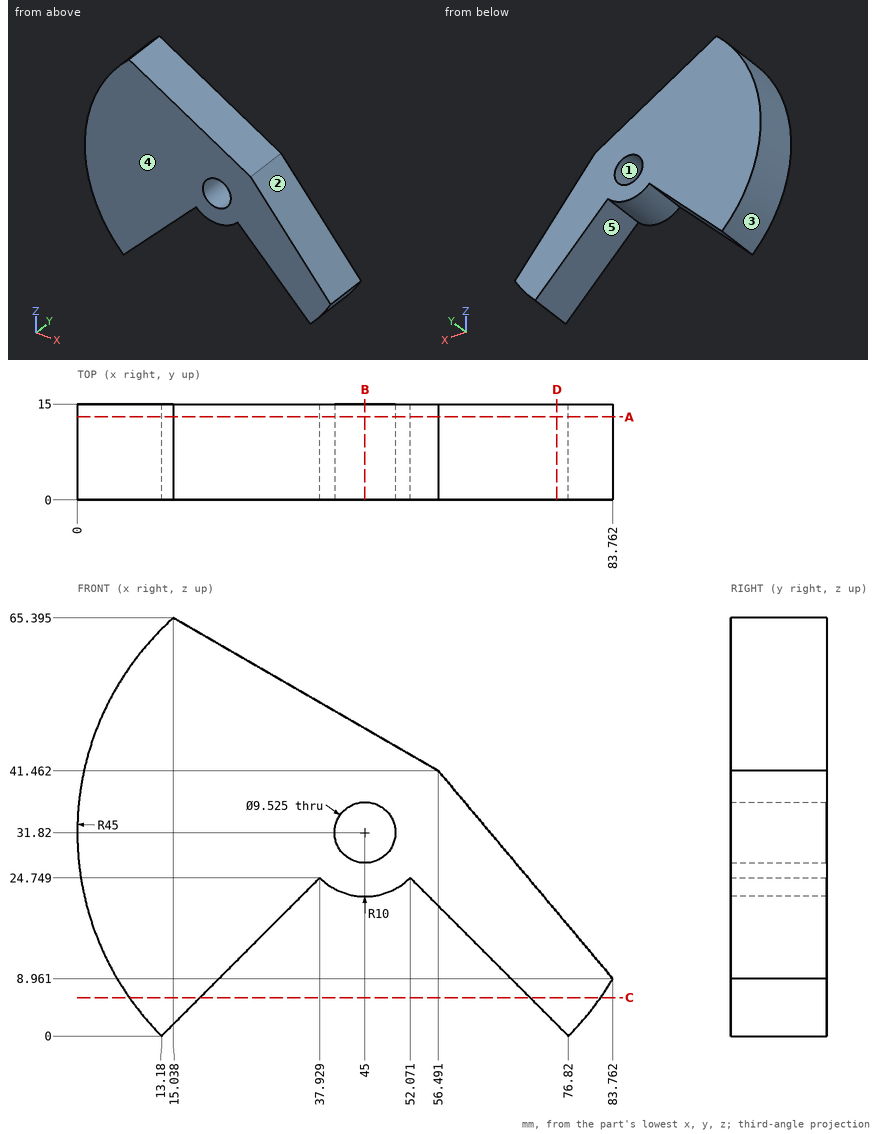
Could you check a few things on this drawing? It's one solid part, dimensions in mm from its lowest x, y, z. A direction names the side the tool comes from. Give positions to 0.01 mm unless a question says otherwise; leave off trailing zeros. Order: outer loops, then holes, each group sorted by start corner. A loop starts at its lowest first (then second) coordinate and runs counter-clockwise, first axis right, second up. Notation, with made-up numbers: M -17.75,17 L 32.25,17 A31 cw 32.25,44 Z; hole C 36.5,45 d1. An arc over 180 degrees is marked long. Use one line per item in the form item = value.
Item 1: If we section it at A-A, the plane y = 13: Write out the boundary of the cut face in (x, z) (1 decimal), and give its area (3 significant figures).
Values follow:
outline = M 13.2,0 L 37.9,24.7 A10 ccw 52.1,24.7 L 76.8,0 A45 ccw 83.8,9 L 56.5,41.5 L 15,65.4 A45 ccw Z; hole C 45,31.8 d9.5
area = 2,570 mm^2
Item 2: Thinking about a two-plate mould opening in X: for the marked faces 1, 2 and 3, which applies, pulls with the +X half, pulls with the -X half, needs draft (parallel to the pull), parting line crosses it, or undercut?
Values follow:
face_1 = undercut
face_2 = pulls with the +X half
face_3 = pulls with the -X half
Item 3: If we section it at D-D, the plane x = 75: Write out the boundary of the cut face in (y, z), and give its area (3 significant figures).
Values follow:
outline = M 0,1.82 L 15,1.82 L 15,19.4 L 0,19.4 Z
area = 264 mm^2
Item 4: Will these pins go through, and if not, where does the flat tip stop? pin 1 Ø3 at (x, y) = (31.5, 7) entering from +Z (1 decimal); pin 2 Ø5 at (y, z) = (5.5, 49.5) entering from +X (1 decimal); pin 3 Ø2 at (x, y) = (20.5, 6.5) entering from +Z.
Values follow:
pin_1 = 56.8
pin_2 = 46.9
pin_3 = 62.82
Item 5: For the marked faces 4 and 5, which set-ups out of +Z, -Z, +X, -X, +Y, -Y let a thin tool reach every point of the face, with its end or its side?
Values follow:
face_4 = +Z, -Z, +X, -X, -Y
face_5 = -Z, +Y, -Y
Item 6: If I drill on line 1 along Z through (x, y) = (45, 4.75) (1 decimal); line 2 along X through (y, z) = (4.25, 21.5); line 3 along X through (y, z) = (2.5, 21), over which ranges is the centre line in solid material (lowest first)? Write a range as [from, to].
Values follow:
line_1 = [21.8, 27.1], [36.6, 48.1]
line_2 = [1.2, 34.68], [55.32, 73.24]
line_3 = [1.32, 34.18], [55.82, 73.66]
Item 7: If we section it at B-B, the plane x = 45: Write out the boundary of the cut face in (y, z) (1 decimal).
Values follow:
outline = M 0,21.8 L 15,21.8 L 15,27.1 L 0,27.1 Z; M 0,36.6 L 15,36.6 L 15,48.1 L 0,48.1 Z
Item 8: If we section it at C-C, the plane z = 6: Write out the boundary of the cut face in (x, y) (1 decimal).
Values follow:
outline = M 8.1,0 L 19.2,0 L 19.2,15 L 8.1,15 Z; M 70.8,0 L 81.9,0 L 81.9,15 L 70.8,15 Z
